Check sheet for the modelled part. Datum: model origin and axes. Units: mm. Face numbers are marked on the shaded views. A direction names the side the tool comes from. Coordinates: 2 decimals unless noted, no trailing zeros. Loops run counter-clockwise (first coordinate to the right, second up) from the corner with the lowest first, then second, coordinate; pieces in that order, holes last.
```python
from build123d import *

# Parameters (mm, degrees)
F0_R     = 4
F0_R_2   = 2
F1_DEPTH = 4
F2_DEPTH = 60
F3_DEPTH = 1


with BuildPart() as f1:
    # F0 (on Top) → F1 (new body)
    with BuildSketch(Plane.XY):
        Circle(F0_R)
        Circle(F0_R_2, mode=Mode.SUBTRACT)
    extrude(amount=-F1_DEPTH)

    # F0 (on Top) → F2 (join)
    with BuildSketch(Plane.XY):
        Circle(F0_R_2)
    extrude(amount=F2_DEPTH)

    # F0 (on Top) → F3 (join)
    with BuildSketch(Plane.XY):
        Circle(F0_R)
        Circle(F0_R_2, mode=Mode.SUBTRACT)
        Circle(F0_R_2)
    extrude(amount=-F3_DEPTH)


solid = f1.part
```
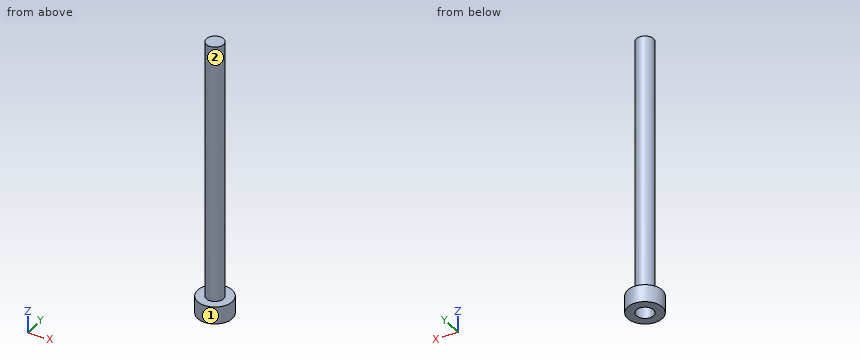
1) Scan lines: line 1 (Y direction, x = 0, z = -2.65); line 2 (Z direction, x = -2, y = 0.5); line 3 (X direction, y = 1, z = 24). Record each from-to range of solid material in increasing order.
Answer sheet:
line 1: y = -4 to -2, 2 to 4
line 2: z = -4 to 0
line 3: x = -1.73 to 1.73
2) Section check A-A on x = 0. Enter the section's corners in (y, z), plus the area to 3 significant figures.
Answer sheet:
outline: (-4, -4) - (-2, -4) - (-2, -1) - (2, -1) - (2, -4) - (4, -4) - (4, 0) - (2, 0) - (2, 60) - (-2, 60) - (-2, 0) - (-4, 0) - close
area: 260 mm2
3) Depth check by flat-ended pin: pin 1 (1.5 mm diameter, centred on x = 0, z = 6, fed in from +Y); pin 2 (4 mm diameter, centred on x = -2, z = 23.5, fed in from -Y); pin 3 (1.5 mm diameter, centred on y = 0, z = 22.5, fed in from -X). Enter the tip coordinate at first touch or a pass-through.
Answer sheet:
pin 1: stops at y = 2
pin 2: stops at y = -2
pin 3: stops at x = -2
4) Section check D-D on x = 3. Enter the section's corners in (y, z), plus the area to 3 significant figures.
Answer sheet:
outline: (-2.65, -4) - (2.65, -4) - (2.65, 0) - (-2.65, 0) - close
area: 21.2 mm2
5) Section check C-C on z = 51.5. Enter the section's corners in (x, y), plus the area to 3 significant figures.
Answer sheet:
outline: circle Ø4 at (0, 0)
area: 12.6 mm2
6) Set-up check for the marked faces 1 and 2: record each of +Z, -Z, +X, -X, +Y, -Y from which the full face is reachable in a straight line by a thin tool's end or side.
Answer sheet:
face 1: +Z, -Z
face 2: +Z
